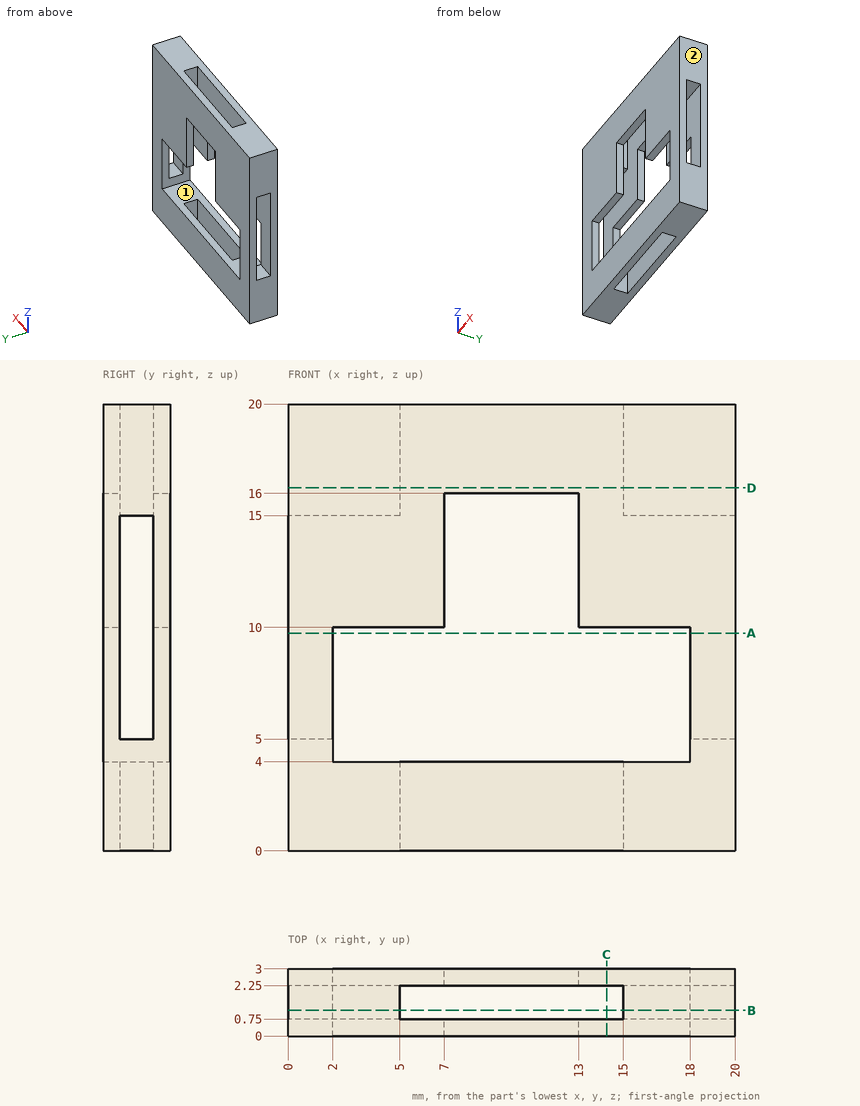
Geometry: see drawing. Coordinates: mm, zero at the bounding-box minimum. A direction names the side the tool comes from. Round coordinates to 2 decimals unless told otherwise and drop trailing zeros. Loops run counter-clockwise (first coordinate to the right, second up) from the corner with the lowest first, then second, coordinate; pieces in that order, holes last. Notation, with made-up numbers: M -16.75,8 L -10.75,8 A10 ccw -10.75,13 Z; hole C -19,68 d8. An arc over 180 degrees is marked long. Use a Markdown table: item, result. Add a question column.
1. Section query B-B on y = 1.15. Return the cut outline in (x, z), then the cut area to 3 significant figures.
2. Contact query for a flat-ended pin moving along its axis: P1, Ø1, axis at y = 1, z = 4.5, coming from the -X side. Output: stop coordinate, or through.
3. Section query A-A on z = 9.75. Return the cut outline in (x, y), then the cut area to 3 significant figures.
4. Section query C-C on x = 14.25. Return the cut outline in (y, z), then the cut area to 3 significant figures.
5. Line query: line 1 (Z direction, x = 1.75, y = 2.1); line 2 (Z direction, x = 11.25, y = 2.55); line 3 (Y direction, x = 17, z = 10.75). Output: solid intervals per line, ascending.
6. Section query D-D on z = 16.25. Return the cut outline in (x, y).
7. Reachability of the marked faces 1 and 2 from +Z, -Z, +X, -X, +Y, -Y: full face, straight path, thin tool, end or side. Return the list, or none.
Reported:
| question | item | result |
|---|---|---|
| 1 | outline | M 0,0 L 5,0 L 5,4 L 2,4 L 2,5 L 0,5 Z; M 0,15 L 5,15 L 5,20 L 0,20 Z; M 15,0 L 20,0 L 20,5 L 18,5 L 18,4 L 15,4 Z; M 15,15 L 20,15 L 20,20 L 15,20 Z |
| 1 | area | 94.0 mm² |
| 2 | P1 | stops at x = 0 |
| 3 | outline | M 0,0 L 2,0 L 2,0.75 L 0,0.75 Z; M 0,2.25 L 2,2.25 L 2,3 L 0,3 Z; M 18,0 L 20,0 L 20,0.75 L 18,0.75 Z; M 18,2.25 L 20,2.25 L 20,3 L 18,3 Z |
| 3 | area | 6.00 mm² |
| 4 | outline | M 0,0 L 0.75,0 L 0.75,4 L 0,4 Z; M 0,10 L 0.75,10 L 0.75,20 L 0,20 Z; M 2.25,0 L 3,0 L 3,4 L 2.25,4 Z; M 2.25,10 L 3,10 L 3,20 L 2.25,20 Z |
| 4 | area | 21.0 mm² |
| 5 | line 1 | z = 0 to 5, 15 to 20 |
| 5 | line 2 | z = 0 to 4, 16 to 20 |
| 5 | line 3 | y = 0 to 0.75, 2.25 to 3 |
| 6 | outline | M 0,0 L 20,0 L 20,3 L 0,3 Z; hole M 5,0.75 L 15,0.75 L 15,2.25 L 5,2.25 Z |
| 7 | face 1 | +Y, -Y |
| 7 | face 2 | +Z, -Z, +X, +Y, -Y |
